Verification items for this drawing (mm, ordinates from the low corner). A direction names the side the tool comes from. Round coordinates to 2 decimals unless told otherwise and drop trailing zeros. Order: outer loops, then holes, each group sorted by start corner. A loop starts at its lowest first (then second) coordinate and runs counter-clockwise, first axis right, second up. Notation, with made-up numbers: (79.5, 28.25) -> (119.5, 28.25) arc R26 ccw to (119.5, 47.25) -> close; hole circle Ø10 at (47.25, 69). An arc over 180 degrees is marked (long way). Return JSON: item names as keys, results as strings. Group by question number.
Item 1: Depth check by flat-ended pin: pin 1 Ø3.5 at (x, z) = (16, 5) entering from -Y. Enter the tip coordinate at first touch or a pass-through.
Item 2: Scan lines: probe 1 along Z at (x, y) = (18.65, 5); probe 2 along Y at (x, z) = (15.75, 5); probe 3 along Y at (x, z) = (13.6, 6.25). Record each from-to range of solid material in increasing order. Write a range as from..to.
Item 3: Sectioned sample at C-C on x = 10. Record the cut outline in (y, z) (1 decimal).
Item 4: Sectioned sample at A-A on y = 5. Give the number of separate pieces and of enclosed holes in the cut face, plus the area to 3 significant figures.
Item 5: Draft check along X on the marked faces 1, 2, 3 and 4. Enter one of: pulls with the +X half, pulls with the -X half, needs draft (parallel to the pull), parting line crosses it, or undercut.
Item 6: Access from +Z, -Z, +X, -X, +Y, -Y to the whole of each face (thin tool, end or side, straight path). Record for the marked faces 5, 6 and 7.
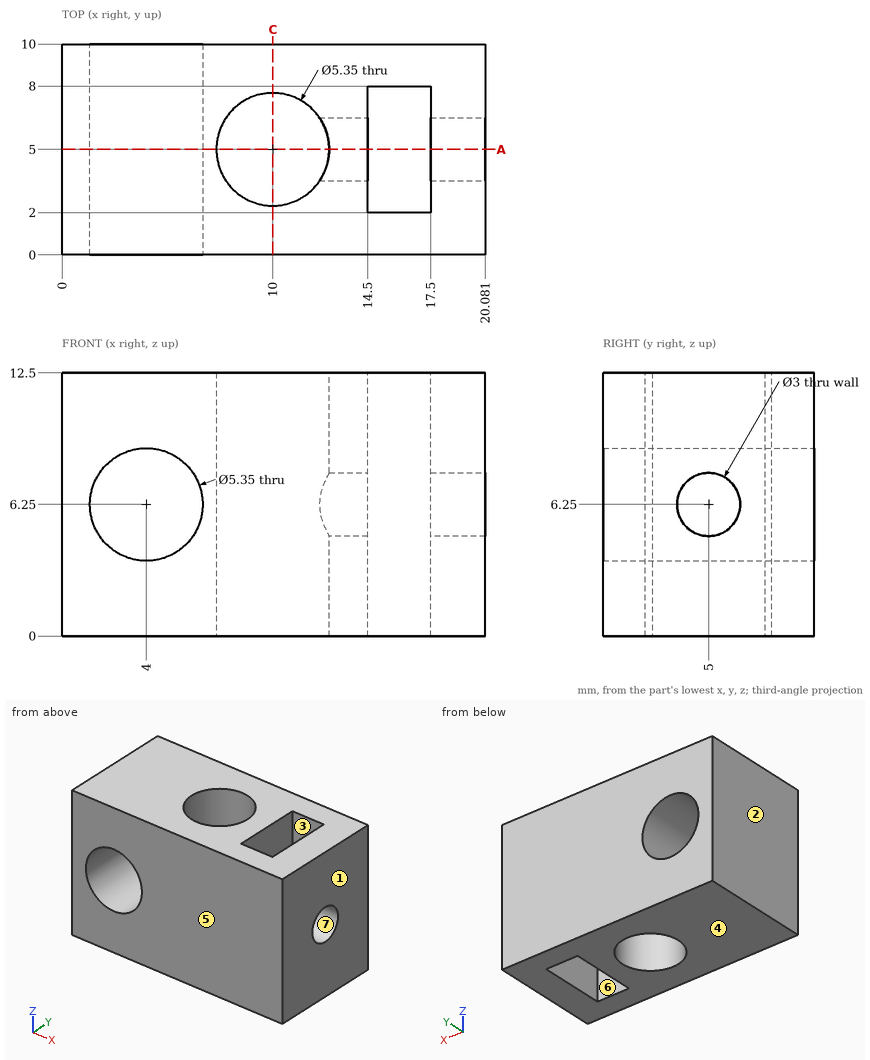
Recorded:
{
 "1": {"pin 1": "y = 0"},
 "2": {"probe 1": "0..4.75, 7.75..12.5", "probe 2": "0..2, 8..10", "probe 3": "0..3.5, 6.5..10"},
 "3": {"outline": "(0, 0) -> (2.3, 0) -> (2.3, 12.5) -> (0, 12.5) -> close; (7.7, 0) -> (10, 0) -> (10, 12.5) -> (7.7, 12.5) -> close"},
 "4": {"separate pieces": "5", "enclosed holes": "1", "area": "111 mm²"},
 "5": {"face 1": "pulls with the +X half", "face 2": "pulls with the -X half", "face 3": "undercut", "face 4": "needs draft"},
 "6": {"face 5": "+Z, -Z, +X, -X, -Y", "face 6": "+Z, -Z", "face 7": "+X"}
}
